Study the drawing (mm; zero at the part's minimum x, y, z) and answer. A direction names the side the tool comes from. Round coordinates to 2 decimals unless told otherwise and drop trailing zeros. Write each loop counter-clockwise with the first axis right and the second up, starting at its lowest first coordinate (ties: lowest second). Pieces come first, ordered by that corner, then holes. Notation, with made-up numbers: M 76,78 L 113,78 A36 ccw 113,116 Z; hole C 22,27 d6. An arc over 180 degrees is marked long. Write each question's results on one line, items separated by ' | '.
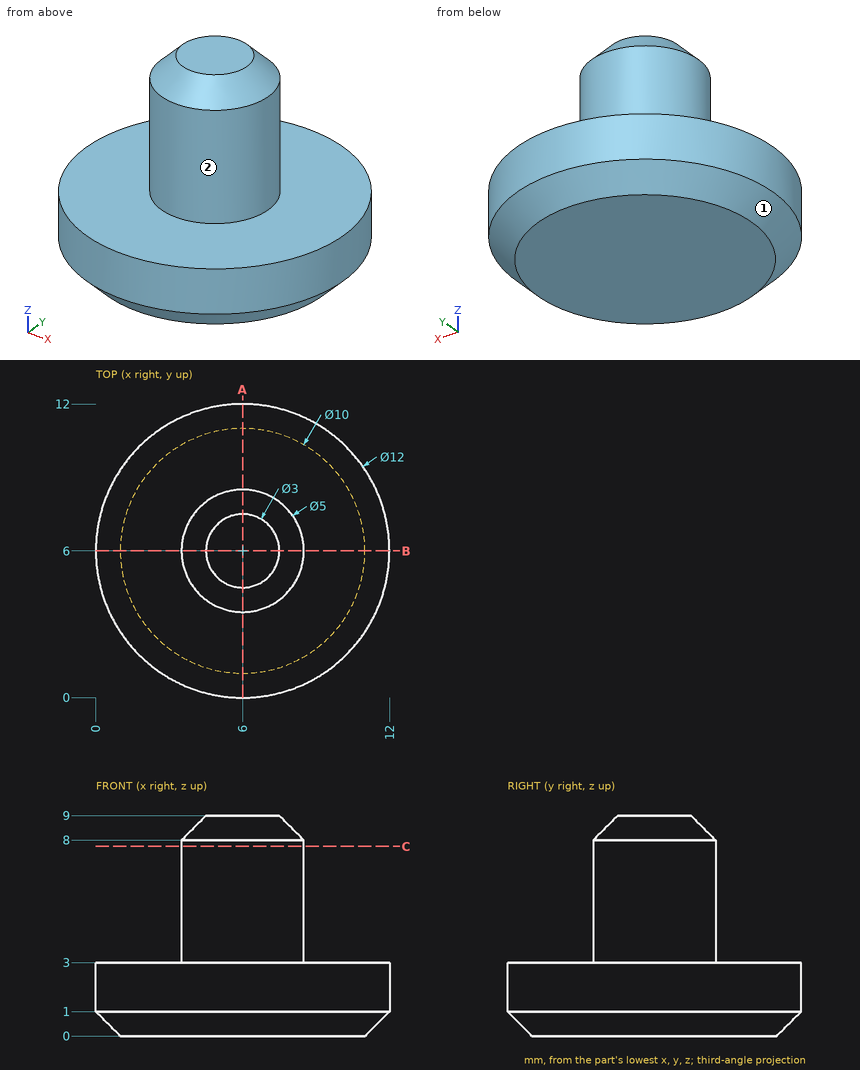
1) Find the intervals of material crossed by line 1 (Z direction, x = 10, y = 6); line 2 (Y direction, x = 8, z = 4); line 3 (Z direction, x = 9.75, y = 9.75), in increasing order.
Return value:
line 1: 0 to 3 | line 2: 4.5 to 7.5 | line 3: 0.3 to 3
2) Each of these flat-tipped pins is pushed along its axis until it touches: pin 1 (3 mm diameter, centred on x = 2.5, y = 6, fed in from +Z); pin 2 (3 mm diameter, centred on x = 10.5, y = 2.5, fed in from +Z); pin 3 (2 mm diameter, centred on y = 5, z = 7.5, fed in from -X); pin 4 (1.5 mm diameter, centred on y = 2.5, z = 7.5, fed in from +X). Where does it stop, or does it pass through?
Return value:
pin 1: z = 8.5 | pin 2: z = 3 | pin 3: x = 3.5 | pin 4: through
3) A tool of negligible diameter and unlimited length cuts with its end or side. For the marked faces 1 and 2, from which of +Z, -Z, +X, -X, +Y, -Y can it reach the whole face along a straight path? Write none if from no direction.
Return value:
face 1: -Z | face 2: +Z
4) Section A-A (x = 6) is taken. Determine the outline of the cut face in (y, z), then the cut area to 3 significant figures.
Return value:
outline: M 0,1 L 1,0 L 11,0 L 12,1 L 12,3 L 8.5,3 L 8.5,8 L 7.5,9 L 4.5,9 L 3.5,8 L 3.5,3 L 0,3 Z | area: 64.0 mm²
5) Section C-C (z = 7.75) is taken. Determine the outline of the cut face in (x, y), then the cut area to 3 significant figures.
Return value:
outline: C 6,6 d5 | area: 19.6 mm²
